Model file for the job. Use its own axes, mm. Give positions to 0.01 mm unless a question says otherwise; leave off trailing zeros. Use CSV: the item, a comma, the result in double quotes. Start each with the question number.
(1) Drop a flat-ended pin along its axis: pin 1 Ø1.8 at (x, z) = (-5.74, -84.37) entering from -Y. Give the stop position or say it passes through.
(2) Band-saw the part on A-A, the plane y = 1.8. Count the separate pieces of the cut face and the enclosed holes in it, then the cut area to 3 significant figures.
(3) Probe L1, parallel to X at y = 2.7, z = 24; L2, parallel to X at y = 0.35, z = -124; L3, parallel to Z at x = -7.75, y = 2.5. List the from-to ranges inside material, lowest first.
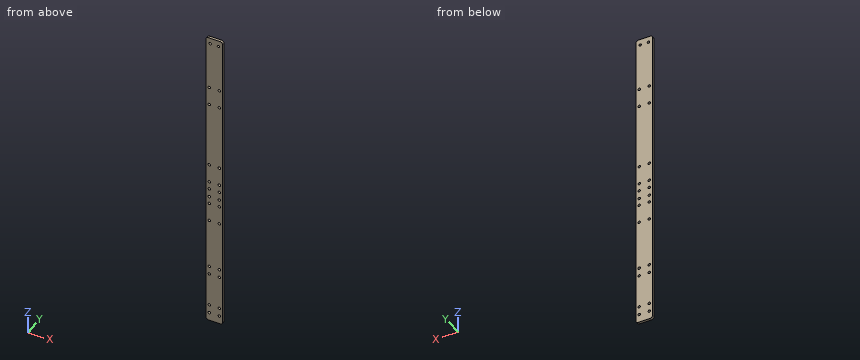
from build123d import *

# Parameters (mm, degrees)
SKETCH_1_W          = 20
SKETCH_1_H          = 510
SKETCH_1_R          = 1.5
EXTRUDE_1_DEPTH     = 3
SKETCH_2_W          = 20
SKETCH_2_H          = 20
CUT_EXTRUDE_1_DEPTH = 257.099704345
SKETCH_3_R          = 1.5
CUT_EXTRUDE_2_DEPTH = 255.347452337
SKETCH_4_W          = 28.97548265
SKETCH_4_H          = 146.861301177
CUT_EXTRUDE_3_DEPTH = 255.347452337
FILLET_1_R          = 3


with BuildPart() as part:
    # 草图1 → 凸台-拉伸1 (new body)
    with BuildSketch(Plane(origin=(0, 0, 0), x_dir=(1, 0, 0), z_dir=(0, 1, 0))):
        with Locations((0.250541192, -0.876894172)):
            Rectangle(SKETCH_1_W, SKETCH_1_H)
        with Locations(Location((5.250541192, -103.876894172, 0), (0, 0, 270))):
            Circle(SKETCH_1_R, mode=Mode.SUBTRACT)
        with Locations(Location((-4.749458808, -103.876894172, 0), (0, 0, 270))):
            Circle(SKETCH_1_R, mode=Mode.SUBTRACT)
        with Locations(Location((6.213384437, -46.87688957, 0), (0, 0, 270))):
            Circle(SKETCH_1_R, mode=Mode.SUBTRACT)
        with Locations(Location((-5.786615563, -46.87688957, 0), (0, 0, 270))):
            Circle(SKETCH_1_R, mode=Mode.SUBTRACT)
        with Locations(Location((6.213384437, -24.87688957, 0), (0, 0, 270))):
            Circle(SKETCH_1_R, mode=Mode.SUBTRACT)
        with Locations(Location((-5.786615563, -24.87688957, 0), (0, 0, 270))):
            Circle(SKETCH_1_R, mode=Mode.SUBTRACT)
        with Locations(Location((6.295138669, 53.123077011, 0), (0, 0, 270))):
            Circle(SKETCH_1_R, mode=Mode.SUBTRACT)
        with Locations(Location((-5.704861331, 53.123077011, 0), (0, 0, 270))):
            Circle(SKETCH_1_R, mode=Mode.SUBTRACT)
        with Locations(Location((6.295138669, 75.123077011, 0), (0, 0, 270))):
            Circle(SKETCH_1_R, mode=Mode.SUBTRACT)
        with Locations(Location((-5.704861331, 75.123077011, 0), (0, 0, 270))):
            Circle(SKETCH_1_R, mode=Mode.SUBTRACT)
        with Locations(Location((6.263384437, 84.37311043, 0), (0, 0, 270))):
            Circle(SKETCH_1_R, mode=Mode.SUBTRACT)
        with Locations(Location((-5.736615563, 84.37311043, 0), (0, 0, 270))):
            Circle(SKETCH_1_R, mode=Mode.SUBTRACT)
        with Locations(Location((6.263384437, 94.37311043, 0), (0, 0, 270))):
            Circle(SKETCH_1_R, mode=Mode.SUBTRACT)
        with Locations(Location((-5.736615563, 94.37311043, 0), (0, 0, 270))):
            Circle(SKETCH_1_R, mode=Mode.SUBTRACT)
        with Locations(Location((6.250541192, 103.123105828, 0), (0, 0, 270))):
            Circle(SKETCH_1_R, mode=Mode.SUBTRACT)
        with Locations(Location((-5.749458808, 103.123105828, 0), (0, 0, 270))):
            Circle(SKETCH_1_R, mode=Mode.SUBTRACT)
        with Locations(Location((6.250541192, 125.123105828, 0), (0, 0, 270))):
            Circle(SKETCH_1_R, mode=Mode.SUBTRACT)
        with Locations(Location((-5.749458808, 125.123105828, 0), (0, 0, 270))):
            Circle(SKETCH_1_R, mode=Mode.SUBTRACT)
        with Locations(Location((6.345138669, 184.373077011, 0), (0, 0, 270))):
            Circle(SKETCH_1_R, mode=Mode.SUBTRACT)
        with Locations(Location((-5.654861331, 184.373077011, 0), (0, 0, 270))):
            Circle(SKETCH_1_R, mode=Mode.SUBTRACT)
        with Locations(Location((6.345138669, 194.373077011, 0), (0, 0, 270))):
            Circle(SKETCH_1_R, mode=Mode.SUBTRACT)
        with Locations(Location((-5.654861331, 194.373077011, 0), (0, 0, 270))):
            Circle(SKETCH_1_R, mode=Mode.SUBTRACT)
        with Locations(Location((6.300541192, 234.373105828, 0), (0, 0, 270))):
            Circle(SKETCH_1_R, mode=Mode.SUBTRACT)
        with Locations(Location((-5.699458808, 234.373105828, 0), (0, 0, 270))):
            Circle(SKETCH_1_R, mode=Mode.SUBTRACT)
        with Locations(Location((6.300541192, 244.373105828, 0), (0, 0, 270))):
            Circle(SKETCH_1_R, mode=Mode.SUBTRACT)
        with Locations(Location((-5.699458808, 244.373105828, 0), (0, 0, 270))):
            Circle(SKETCH_1_R, mode=Mode.SUBTRACT)
    extrude(amount=EXTRUDE_1_DEPTH)

    # 草图2 → 切除-拉伸1 (cut, through all)
    with BuildSketch(Plane(origin=(0, 3, 0), x_dir=(1, 0, 0), z_dir=(0, 1, 0))):
        with Locations((0.250541192, -245.876894172)):
            Rectangle(SKETCH_2_W, SKETCH_2_H)
    extrude(amount=-CUT_EXTRUDE_1_DEPTH, mode=Mode.SUBTRACT)

    # 草图3 → 切除-拉伸2 (cut, through all)
    with BuildSketch(Plane(origin=(0, 3, 0), x_dir=(1, 0, 0), z_dir=(0, 1, 0))):
        with Locations(Location((-5.749458808, -170.876894172, 0), (0, 0, 270))):
            Circle(SKETCH_3_R)
        with Locations(Location((-5.749458808, -200.876894172, 0), (0, 0, 270))):
            Circle(SKETCH_3_R)
        with Locations(Location((6.250541192, -170.876894172, 0), (0, 0, 90))):
            Circle(SKETCH_3_R)
        with Locations(Location((6.250541192, -200.876894172, 0), (0, 0, 90))):
            Circle(SKETCH_3_R)
    extrude(amount=-CUT_EXTRUDE_2_DEPTH, mode=Mode.SUBTRACT)

    # 草图4 → 切除-拉伸3 (cut, through all)
    with BuildSketch(Plane(origin=(0, 3, 0), x_dir=(1, 0, 0), z_dir=(0, 1, 0))):
        with Locations((4.738282517, -184.307544761)):
            Rectangle(SKETCH_4_W, SKETCH_4_H)
    extrude(amount=-CUT_EXTRUDE_3_DEPTH, mode=Mode.SUBTRACT)

    # 圆角1
    fillet_1_edges = [part.edges().sort_by_distance(p)[0] for p in [
        (10.250541192, 1.5, 110.876894172),
        (-9.749458808, 1.5, 110.876894172),
        (10.250541192, 1.5, -254.123105828),
        (-9.749458808, 1.5, -254.123105828),
    ]]
    fillet(fillet_1_edges, radius=FILLET_1_R)


solid = part.part
Answer block:
1,pin 1,"passes through"
2,separate pieces,"1"
2,enclosed holes,"26"
2,area,"7,110 mm2"
3,L1,"x = -9.75 to -7, -4.57 to 5, 7.43 to 10.25"
3,L2,"x = -9.75 to -6.74, -4.76 to 5.26, 7.24 to 10.25"
3,L3,"z = -253.95 to 110.71"
